Part model, mm, in its own coordinate system. Face numbers are marked on the shaded views. A direction names the side the tool comes from. Give positions to 0.01 mm unless a question says otherwise; leave off trailing zeros. Write each loop counter-clockwise with the first axis right and the second up, starting at its lowest first coordinate (ties: lowest second). Pieces come first, ordered by that corner, then holes. Notation, with made-up numbers: (-38.5, 47) - (-12.5, 47) arc R16 ccw to (-12.5, 71) - close; hole circle Ø10 at (-15.5, -21.5). An arc over 180 degrees is marked (long way). Answer as a JSON object with one key per item and string values. Group by question number.
```python
from build123d import *

# Parameters (mm, degrees)
F1_DEPTH = 38.1
F2_DEPTH = 12.7
F0_W     = 22.1240029774
F0_H     = 19.05
F0_H_2   = 5.4648819111
F0_H_3   = 3.4845191814
F3_DEPTH = 25.4
F4_R     = 6.35


with BuildPart() as f1:
    # F0 (on Front) → F1 (new body, symmetric)
    with BuildSketch(Plane.XZ):
        Polygon((48.99266572, -19.2026612566), (68.04266572, -19.2026612566), (68.04266572, 19.2026612566), (-68.04266572, 19.2026612566), (-68.04266572, -19.2026612566), align=None)
    extrude(amount=F1_DEPTH, both=True)

    # F0 (on Front) → F2 (join, symmetric)
    with BuildSketch(Plane.XZ):
        with BuildLine():
            Line((48.99266572, -44.1608317196), (48.99266572, -19.2026612566))
            Line((48.99266572, -19.2026612566), (-68.04266572, -19.2026612566))
            add(Edge.make_bspline(
                [(-68.04266572, -19.2026612566), (-17.0981840349, -23.8250708772), (13.6489767473, -70.337126404), (75.1989668614, -74.6391754041)],
                knots=[0, 0, 0, 0, 154.432294088, 154.432294088, 154.432294088, 154.432294088], degree=3))
            ThreePointArc((75.1989668614, -74.6391754041), (56.4450578335, -64.258715024), (48.99266572, -44.1608317196))
        make_face()
        with BuildLine():
            Line((68.04266572, -44.1608317196), (68.04266572, -19.2026612566))
            Line((68.04266572, -19.2026612566), (48.99266572, -19.2026612566))
            Line((48.99266572, -19.2026612566), (48.99266572, -44.1608317196))
            ThreePointArc((48.99266572, -44.1608317196), (56.4450578335, -64.258715024), (75.1989668614, -74.6391754041))
            add(Edge.make_bspline(
                [(75.1989668614, -74.6391754041), (77.3256902061, -74.7878231622), (79.4891888852, -74.8860766175), (81.6915667764, -74.930466459)],
                knots=[154.432294088, 154.432294088, 154.432294088, 154.432294088, 159.7683593643, 159.7683593643, 159.7683593643, 159.7683593643], degree=3))
            Line((81.6915667764, -74.930466459), (85.9540551901, -74.930466459))
            Line((85.9540551901, -74.930466459), (85.9540551901, -55.880466459))
            Line((85.9540551901, -55.880466459), (80.9756178971, -55.880466459))
            ThreePointArc((80.9756178971, -55.880466459), (71.9113494041, -52.8873873179), (68.04266572, -44.1608317196))
        make_face()
    extrude(amount=F2_DEPTH, both=True)

    # F0 (on Front) → F3 (join, symmetric)
    with BuildSketch(Plane.XZ):
        Polygon((108.0780581675, -52.3959472775), (108.0780581675, -55.880466459), (108.0780581675, -74.930466459), (108.0780581675, -80.3953483701), (148.1291949749, -80.3953483701), (148.1291949749, -52.3959472775), align=None)
        with Locations((97.0160566788, -65.405466459)):
            Rectangle(F0_W, F0_H)
        with Locations((97.0160566788, -77.6629074145)):
            Rectangle(F0_W, F0_H_2)
        with Locations((97.0160566788, -54.1382068683)):
            Rectangle(F0_W, F0_H_3)
    extrude(amount=F3_DEPTH, both=True)

    # F4
    f4_edges = [f1.edges().sort_by_distance(p)[0] for p in [
        (68.042666, -38.1, 0),
        (-68.042666, -38.1, 0),
        (-68.042666, 38.1, 0),
        (68.042666, 38.1, 0),
    ]]
    fillet(f4_edges, radius=F4_R)


solid = f1.part
```
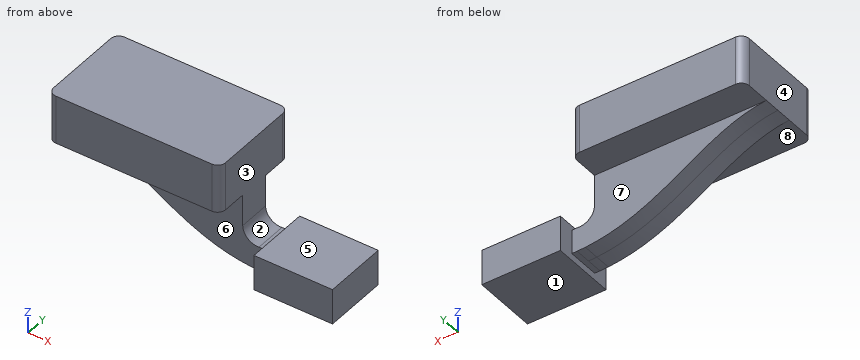
1) Drop flat-ended pins along their axis: P1, Ø1.5, axis at x = 83.5, y = 0, coming from the +Z side; P2, Ø8.5, axis at x = 107.5, z = -73, coming from the +Y side; P3, Ø1.5, axis at y = 16.5, z = -1.5, coming from the +X side; P4, Ø16.5, axis at x = -12.5, z = -53, coming from the -Y side. Give the stop position or say it passes through.
2) Drill centre lines: line 1 along X through (y, z) = (-16, -71.5); line 2 along X through (y, z) = (21, -4.5); line 3 along Z through (x, y) = (-54, -20). Where is each one in solid material? Low to high. Write a range as from..to.
3) Which spindle directions (+Z, -Z, +X, -X, +Y, -Y) get a long thin tool onto all of the face, cutting with end or side? Do the marked faces 5, 6, 7 and 8. Say none if no direction does.
4) Saw through at A-A (y = 22.5). List the corners of the cut face in (x, z), and give its area (3 significant figures).
5) Saw through at B-B (z = 3.5). List the corners of the cut face in (x, y).
6) Two-plate mould, pull along X, no slides. Class the marked faces 1, 2, 3 and 4: +X half, -X half, draft (parallel to the pull), parting line (faces both ways), or undercut.
7) Saw through at C-C (x = 99). List the corners of the cut face in (y, z), and give its area (3 significant figures).
Checks:
{
 "1": {"P1": "z = -55.88", "P2": "y = 25.4", "P3": "x = 68.04", "P4": "through"},
 "2": {"line 1": "85.95..148.13", "line 2": "-68.04..68.04", "line 3": "-19.2..19.2"},
 "3": {"face 5": "+Z, +X, +Y, -Y", "face 6": "-Z, -X, -Y", "face 7": "-Z, -X, +Y", "face 8": "-Z, +X, -X, -Y"},
 "4": {"outline": "(-68.04, -19.2) - (68.04, -19.2) - (68.04, 19.2) - (-68.04, 19.2) - close; (85.95, -80.4) - (148.13, -80.4) - (148.13, -52.4) - (85.95, -52.4) - close", "area": "6,970 mm2"},
 "5": {"outline": "(-68.04, -31.75) arc R6.35 ccw to (-61.69, -38.1) - (61.69, -38.1) arc R6.35 ccw to (68.04, -31.75) - (68.04, 31.75) arc R6.35 ccw to (61.69, 38.1) - (-61.69, 38.1) arc R6.35 ccw to (-68.04, 31.75) - close"},
 "6": {"face 1": "draft", "face 2": "undercut", "face 3": "+X half", "face 4": "-X half"},
 "7": {"outline": "(-25.4, -80.4) - (25.4, -80.4) - (25.4, -52.4) - (-25.4, -52.4) - close", "area": "1,420 mm2"}
}
